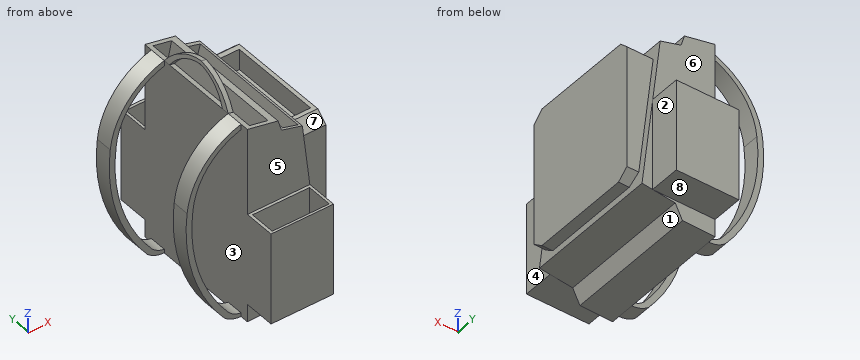
```python
from build123d import *

# Parameters (mm, degrees)
F1_DEPTH  = 330.2
F3_DEPTH  = 203.2
F4_W      = 41.5566265583
F4_H      = 483.5203289986
F5_DEPTH  = 139.7
F8_DEPTH  = 304.8
F9_DEPTH  = 304.8
F13_DEPTH = 50.8
F14_DEPTH = 50.8
F15_DEPTH = 50.8
F16_W     = 12.4509147432
F16_H     = 205.8088108897
F17_DEPTH = 60.96
F19_DEPTH = 25.4
F20_DEPTH = 25.4
F21_W     = 153.1679212224
F21_H     = 225.7029655442
F22_DEPTH = 76.2
F23_W     = 153.0837979386
F23_H     = 225.7128436606
F24_DEPTH = 76.2
F25_W     = 139.6465194412
F25_H     = 63.5316371918
F26_DEPTH = 76.2
F27_W     = 140.8935589716
F27_H     = 64.2704893835
F28_DEPTH = 76.2


with BuildPart() as f1:
    # F0 (on Front) → F1 (new body)
    with BuildSketch(Plane.XZ):
        Polygon((75.0250443816, 274.7305631638), (0, 290.2742098035), (0, -192.3257901965), (80.0467804074, -190.855011344), (97.7545654154, -155.2051532254), (179.0464967489, -145.659506321), (134.568348527, 233.1220060587), (83.6337208748, 247.4697828293), align=None)
    extrude(amount=F1_DEPTH)

    # F2 (on Right) → F3 (join)
    with BuildSketch(Plane.YZ):
        Polygon((-36.8141271174, 215.1695936918), (-289.5758748055, 216.376081109), (-316.1188662052, 192.8493380547), (-316.1188662052, -106.9659143686), (-290.7823622227, -126.2699067593), (-44.0531261265, -126.2699067593), (-16.9068686664, -104.5529171824), (-16.9068686664, 195.8655864), align=None)
    extrude(amount=F3_DEPTH)

    # F4 (on Right) → F5 (join)
    with BuildSketch(Plane.YZ):
        Polygon((-20.9644548595, -191.9956207275), (-20.9644548595, 291.524708271), (-62.5730231404, 291.524708271), (-62.5730231404, -191.9956207275), (-26.7035681754, -191.9956207275), align=None)
        with Locations((-289.1601473093, 49.7645437717)):
            Rectangle(F4_W, F4_H)
    extrude(amount=-F5_DEPTH)

    # F7 (on face) → F8 (cut)
    with BuildSketch(Plane(origin=(0, -20.9644548595, 0), x_dir=(-1, 0, 0), z_dir=(0, 1, 0))):
        with BuildLine():
            Line((0, 291.524708271), (0, 290.2742098035))
            ThreePointArc((0, 290.2742098035), (90.3834546734, 230.8148027656), (132.1892142296, 131.0306936502))
            ThreePointArc((132.1892142296, 131.0306936502), (117.5430207962, -31.2395021377), (41.5639653802, -175.3689944744))
            ThreePointArc((41.5639653802, -175.3689944744), (22.3830735082, -187.6847842501), (0, -191.9956207275))
            Line((0, -191.9956207275), (139.7, -191.9956207275))
            Line((139.7, -191.9956207275), (139.7, 291.524708271))
            Line((139.7, 291.524708271), (0, 291.524708271))
        make_face()
    extrude(amount=-F8_DEPTH, mode=Mode.SUBTRACT)

    # F7 (on face) → F9 (cut)
    with BuildSketch(Plane(origin=(0, -20.9644548595, 0), x_dir=(-1, 0, 0), z_dir=(0, 1, 0))):
        with BuildLine():
            ThreePointArc((30.8481585234, -166.6212230921), (104.4091983221, -26.9422304703), (117.9412454367, 130.3420066833))
            ThreePointArc((117.9412454367, 130.3420066833), (81.3233643675, 221.5363124881), (0, 276.7067849636))
            Line((0, 276.7067849636), (0, -182.9511970282))
            ThreePointArc((0, -182.9511970282), (16.9048608228, -177.5834823958), (30.8481585234, -166.6212230921))
        make_face()
    extrude(amount=-F9_DEPTH, mode=Mode.SUBTRACT)

    # F12 (on face) → F13 (cut)
    with BuildSketch(Plane(origin=(0, 1.026189658, 214.9889735368), x_dir=(1, 0, 0), z_dir=(0, 0.0047731656, 0.9999886084))):
        Polygon((193.5474094368, -50.5835317066), (145.7960009575, -50.5567677319), (144.2719995975, -50.5567677319), (144.2719995975, -280.1753878593), (193.5474094368, -280.1753878593), align=None)
    extrude(amount=-F13_DEPTH, mode=Mode.SUBTRACT)

    # F10 (on face) → F14 (cut)
    with BuildSketch(Plane(origin=(57.6637293587, 0, 278.3274706783), x_dir=(0.9792054246, 0, -0.202871231), z_dir=(0.202871231, 0, 0.9792054246))):
        Polygon((0, -10.4822274297), (-44.3622209132, -10.4822274297), (-46.4373715222, -10.4822274297), (-46.4373715222, -320.8020031452), (0, -320.8020031452), align=None)
    extrude(amount=-F14_DEPTH, mode=Mode.SUBTRACT)

    # F11 (on face) → F15 (cut)
    with BuildSketch(Plane(origin=(70.7334014159, 0, 251.1036741994), x_dir=(0.9625404698, 0, -0.2711380534), z_dir=(0.2711380534, 0, 0.9625404698))):
        Polygon((60.0396618247, -9.9059985951), (20.4569026828, -9.9059985951), (21.5124394745, -323.8500058651), (60.0396618247, -323.8500058651), align=None)
    extrude(amount=-F15_DEPTH, mode=Mode.SUBTRACT)

    # F16 (on face) → F17 (join)
    with BuildSketch(Plane(origin=(57.6637293587, 0, 278.3274706783), x_dir=(0.9792054246, 0, -0.202871231), z_dir=(0.202871231, 0, 0.9792054246))):
        with Locations((-52.6628288938, -165.4774285853)):
            Rectangle(F16_W, F16_H)
    extrude(amount=F17_DEPTH)

    # F18 (on face) → F19 (cut)
    with BuildSketch(Plane(origin=(-57.6637293587, 0, 11.9467391251), x_dir=(0, -1, 0), z_dir=(-0.9792054246, 0, 0.202871231))):
        with BuildLine():
            ThreePointArc((62.5730231404, 284.2380808719), (106.8196773219, 326.8815108015), (165.4774285853, 345.1980808719))
            Line((165.4774285853, 345.1980808719), (62.5730231404, 345.1980808719))
            Line((62.5730231404, 345.1980808719), (62.5730231404, 284.2380808719))
        make_face()
        with BuildLine():
            Line((268.3818340302, 345.1980808719), (165.4774285853, 345.1980808719))
            ThreePointArc((165.4774285853, 345.1980808719), (223.2646342428, 325.4119737611), (268.3818340302, 284.2380808719))
            Line((268.3818340302, 284.2380808719), (268.3818340302, 345.1980808719))
        make_face()
    extrude(amount=-F19_DEPTH, mode=Mode.SUBTRACT)

    # F18 (on face) → F20 (cut)
    with BuildSketch(Plane(origin=(-57.6637293587, 0, 11.9467391251), x_dir=(0, -1, 0), z_dir=(-0.9792054246, 0, 0.202871231))):
        with BuildLine():
            ThreePointArc((165.4774285853, 337.3909592628), (115.9669465301, 321.2480632926), (79.3316885829, 284.2380808719))
            Line((79.3316885829, 284.2380808719), (249.7253417969, 284.2380808719))
            ThreePointArc((249.7253417969, 284.2380808719), (213.6637620757, 320.4234559725), (165.4774285853, 337.3909592628))
        make_face()
    extrude(amount=-F20_DEPTH, mode=Mode.SUBTRACT)

    # F21 (on face) → F22 (join)
    with BuildSketch(Plane(origin=(0, 0, 0), x_dir=(-1, 0, 0), z_dir=(0, 1, 0))):
        with Locations((-76.5839606112, -35.8467967741)):
            Rectangle(F21_W, F21_H)
    extrude(amount=F22_DEPTH)

    # F23 (on face) → F24 (join)
    with BuildSketch(Plane.XZ.offset(330.2)):
        with Locations((76.5418989693, -35.8517358323)):
            Rectangle(F23_W, F23_H)
    extrude(amount=F24_DEPTH)

    # F25 (on face) → F26 (cut)
    with BuildSketch(Plane.XY.offset(77.004685998)):
        with Locations((77.0478153136, -368.982732296)):
            Rectangle(F25_W, F25_H)
    extrude(amount=-F26_DEPTH, mode=Mode.SUBTRACT)

    # F27 (on face) → F28 (cut)
    with BuildSketch(Plane.XY.offset(77.004685998)):
        with Locations((76.6873457469, 37.3120044824)):
            Rectangle(F27_W, F27_H)
    extrude(amount=-F28_DEPTH, mode=Mode.SUBTRACT)


solid = f1.part
```
Read the model definition and answer for the solid it produces. Units are mm, in the model's axes. Face numbers are marked on the shaded views. A direction names the side the tool comes from. Coordinates: 2 decimals unless noted, no trailing zeros. Write each loop counter-clockwise with the first axis right and the second up, starting at its lowest first coordinate (ties: lowest second). Pieces come first, ordered by that corner, then holes. Notation, with made-up numbers: (-28.5, -35.5) -> (1.5, -35.5) arc R27 cw to (1.5, -3.5) -> close; hole circle Ø2 at (76.25, 20). An arc over 180 degrees is marked (long way). Answer as a JSON object with one key per item and string values.
Q1. The part is cut by section C-C on x = -80. Give the vertices of the cut face in (y, z), then the cut area to 3 significant figures.
The answers:
{"outline": "(-309.94, -119.27) -> (-268.38, -119.27) -> (-268.38, -89.86) -> (-309.94, -89.86) -> close; (-309.94, 223.16) -> (-268.38, 223.16) -> (-268.38, 242.31) -> (-309.94, 242.31) -> close; (-62.57, -119.27) -> (-20.96, -119.27) -> (-20.96, -89.86) -> (-62.57, -89.86) -> close; (-62.57, 223.16) -> (-20.96, 223.16) -> (-20.96, 242.31) -> (-62.57, 242.31) -> close", "area": "4,040 mm2"}
Q2. The part is cut by section B-B on y = -348.5. Give the vertices of the cut face in (x, z), then the cut area to 3 significant figures.
The answers:
{"outline": "(0, -148.71) -> (153.08, -148.71) -> (153.08, 77) -> (146.87, 77) -> (146.87, 0.8) -> (7.22, 0.8) -> (7.22, 77) -> (0, 77) -> close", "area": "23,900 mm2"}
Q3. The part is cut by section A-A on z = 44.5. Give the vertices of the cut face in (x, y).
The answers:
{"outline": "(-132.46, -309.94) -> (-118.43, -309.94) -> (-118.43, -268.38) -> (-132.46, -268.38) -> close; (-132.46, -62.57) -> (-118.43, -62.57) -> (-118.43, -20.96) -> (-132.46, -20.96) -> close; (0, -406.4) -> (153.08, -406.4) -> (153.08, -330.2) -> (156.72, -330.2) -> (156.72, -316.12) -> (203.2, -316.12) -> (203.2, -16.91) -> (156.72, -16.91) -> (156.72, 0) -> (153.17, 0) -> (153.17, 76.2) -> (0, 76.2) -> close; hole (6.24, 5.18) -> (147.13, 5.18) -> (147.13, 69.45) -> (6.24, 69.45) -> close; hole (7.22, -400.75) -> (146.87, -400.75) -> (146.87, -337.22) -> (7.22, -337.22) -> close"}
Q4. Flat-ended cylindrical pins translate along their axes: pin 1 Ø5 at (y, z) = (-222, 224.5) entering from +X; pin 2 Ø5 at (x, z) = (118.5, 140) entering from -Y; pin 3 Ø2 at (x, y) = (-65.5, -293) entering from -Z. Find the tip coordinate at first contact, or state that the pin passes through.
The answers:
{"pin 1": "stops at x = 135.87", "pin 2": "stops at y = -330.2", "pin 3": "stops at z = -144.32"}
Q5. Consider line 1 (X direction, y = -339, z = 10); line 2 (Y direction, x = -105.5, z = -26); line 3 (X direction, y = -261, z = 148). Determine where each line is inside the solid, lowest interval first. Write a range as [from, to].
The answers:
{"line 1": "x = [0, 7.22], [146.87, 153.08]", "line 2": "y = [-309.94, -268.38], [-62.57, -20.96]", "line 3": "x = [0, 203.2]"}
Q6. A tool of negligible diameter and unlimited length cuts with its end or side. For the marked faces 4, 5, 6, 7 and 8, from which of +Z, -Z, +X, -X, +Y, -Y can it reach the whole face along a straight path? Write none if from no direction.
The answers:
{"face 4": "+Z, -Z, +X, -Y", "face 5": "+Z, +X, -X, -Y", "face 6": "+Z, +X, -X, +Y", "face 7": "+Z, +X, -Y", "face 8": "-Z, +X, -X, +Y"}
Q7. Determine the mould class of the marked faces 1, 2 and 3 for opening direction Z: pulls with the +Z half, pulls with the -Z half, needs draft (parallel to the pull), parting line crosses it, or undercut.
The answers:
{"face 1": "pulls with the -Z half", "face 2": "needs draft", "face 3": "undercut"}
Q8. The part is cut by section D-D on z = 267. Give the vertices of the cut face in (x, y), then the cut area to 3 significant figures.
The answers:
{"outline": "(-50.06, -309.94) -> (-24.45, -309.94) -> (-24.45, -268.38) -> (-50.06, -268.38) -> close; (-50.06, -62.57) -> (-24.45, -62.57) -> (-24.45, -20.96) -> (-50.06, -20.96) -> close; (0, -330.2) -> (77.47, -330.2) -> (77.47, 0) -> (0, 0) -> close; hole (7.89, -320.8) -> (55.32, -320.8) -> (55.32, -10.48) -> (7.89, -10.48) -> close", "area": "13,000 mm2"}
